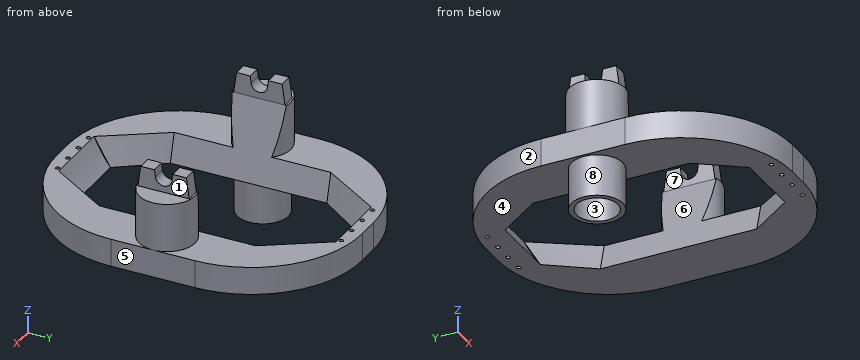
```python
from build123d import *

# Parameters (mm, degrees)
SKETCH_1_R                      = 18.5
SKETCH_1_R_2                    = 15
EXTRUDE_1_DEPTH                 = 30
SKETCH_2_R                      = 20.2
SKETCH_2_R_2                    = 15
EXTRUDE_2_DEPTH                 = 5
SKETCH_3_R                      = 20.2
EXTRUDE_3_DEPTH                 = 50
EXTRUDE_4_DEPTH                 = 5
EXTRUDE_5_DEPTH                 = 20
FILLET_1_R                      = 80
CUT_EXTRUDE_2_REACH             = 174.924
SKETCH_7_R                      = 110
CUT_EXTRUDE_2_DIRECTION_2_REACH = 174.924
SKETCH_11_R                     = 1.5
CUT_EXTRUDE_3_DEPTH             = 25
SKETCH_12_W                     = 57.061720969
SKETCH_12_H                     = 113.011504976
CUT_EXTRUDE_4_DEPTH             = 20


with BuildPart() as part:
    # 草图1 → 凸台-拉伸1 (new body)
    with BuildSketch(Plane.XY):
        Circle(SKETCH_1_R)
        Circle(SKETCH_1_R_2, mode=Mode.SUBTRACT)
    extrude(amount=EXTRUDE_1_DEPTH)

    # 草图2 → 凸台-拉伸2 (add)
    with BuildSketch(Plane.XY.offset(30)):
        Circle(SKETCH_2_R)
        Circle(SKETCH_2_R_2, mode=Mode.SUBTRACT)
    extrude_2 = extrude(amount=EXTRUDE_2_DEPTH)

    # 草图3 → 凸台-拉伸3 (add)
    with BuildSketch(Plane.XY.offset(35)):
        Circle(SKETCH_3_R)
    extrude_3 = extrude(amount=EXTRUDE_3_DEPTH)

    # 草图5 → 凸台-拉伸4 (add, symmetric)
    with BuildSketch(Plane(origin=(0, 0, 0), x_dir=(0, -1, 0), z_dir=(1, 0, 0))):
        with BuildLine():
            Line((-18.5, -85), (18.5, -85))
            Line((18.5, -85), (16.5, -100))
            Line((16.5, -100), (6.5, -100))
            Line((6.5, -100), (5.966081527, -95))
            ThreePointArc((5.966081527, -95), (0, -89.637080228), (-5.966081527, -95))
            Line((-5.966081527, -95), (-6.5, -100))
            Line((-6.5, -100), (-16.5, -100))
            Line((-16.5, -100), (-18.5, -85))
        make_face()
    extrude_4 = extrude(amount=EXTRUDE_4_DEPTH, both=True)

    # 草图6 → 凸台-拉伸5 (add)
    with BuildSketch(Plane(origin=(0, 0, 30), x_dir=(-1, 0, 0), z_dir=(0, 0, -1))):
        Polygon((20.2, 0), (20.2, 110.346509277), (-155.6, 110.346509277), (-155.6, 0), (-155.6, -110.346509277), (20.2, -110.346509277), align=None)
        Polygon((-115.2, 56.505752488), (-92.7, 56.505752488), (-92.7, 85), (-42.7, 85), (-42.7, 56.505752488), (-20.2, 56.505752488), (-20.2, -56.505752488), (-42.7, -56.505752488), (-42.7, -85), (-92.7, -85), (-92.7, -56.505752488), (-115.2, -56.505752488), align=None, mode=Mode.SUBTRACT)
    extrude(amount=-EXTRUDE_5_DEPTH)

    # 镜向1: 凸台-拉伸2, 凸台-拉伸3, 凸台-拉伸4 across plane
    add(extrude_2.mirror(Plane.ZY.offset(-67.7)))
    add(extrude_3.mirror(Plane.ZY.offset(-67.7)))
    add(extrude_4.mirror(Plane.ZY.offset(-67.7)))

    # 圆角1
    fillet_1_edges = [part.edges().sort_by_distance(p)[0] for p in [
        (-20.2, 110.346509277, 40),
        (-20.2, -110.346509277, 40),
        (155.6, -110.346509277, 40),
        (155.6, 110.346509277, 40),
    ]]
    fillet(fillet_1_edges, radius=FILLET_1_R)

    # 切除-拉伸2: up to this face of the body (flat: up to its plane)
    cut_extrude_2_end = Plane(part.part.faces().sort_by_distance((42.7, 70.752876244, 40))[0])
    # 草图7 → 切除-拉伸2 (cut, up to the picked face)
    with BuildSketch(Plane(origin=(67.7, 0, 0), x_dir=(0, 0, -1), z_dir=(1, 0, 0)), mode=Mode.PRIVATE) as cut_extrude_2_sk1:
        with Locations((-95.637080228, 0)):
            Circle(SKETCH_7_R)
    cut_extrude_2_tool1 = split(extrude(cut_extrude_2_sk1.sketch, amount=-CUT_EXTRUDE_2_REACH, mode=Mode.PRIVATE), bisect_by=cut_extrude_2_end, keep=Keep.BOTH, mode=Mode.PRIVATE)
    add(cut_extrude_2_tool1.solids().sort_by(Axis((67.7, 0, 95.63708), (-1, 0, 0)))[0], mode=Mode.SUBTRACT)

    # 切除-拉伸2 direction 2: up to this face of the body (flat: up to its plane)
    cut_extrude_2_direction_2_end = Plane(part.part.faces().sort_by_distance((92.7, 70.752876244, 40))[0])
    # 草图7 → 切除-拉伸2 direction 2 (cut, up to the picked face)
    with BuildSketch(Plane(origin=(67.7, 0, 0), x_dir=(0, 0, -1), z_dir=(1, 0, 0)), mode=Mode.PRIVATE) as cut_extrude_2_direction_2_sk1:
        with Locations((-95.637080228, 0)):
            Circle(SKETCH_7_R)
    cut_extrude_2_direction_2_tool1 = split(extrude(cut_extrude_2_direction_2_sk1.sketch, amount=CUT_EXTRUDE_2_DIRECTION_2_REACH, mode=Mode.PRIVATE), bisect_by=cut_extrude_2_direction_2_end, keep=Keep.BOTH, mode=Mode.PRIVATE)
    add(cut_extrude_2_direction_2_tool1.solids().sort_by(Axis((67.7, 0, 95.63708), (1, 0, 0)))[0], mode=Mode.SUBTRACT)

    # 草图11 → 切除-拉伸3 (cut)
    with BuildSketch(Plane(origin=(0, 0, 30), x_dir=(-1, 0, 0), z_dir=(0, 0, -1))):
        with Locations((-89.646136586, -102.489523561)):
            Circle(SKETCH_11_R)
        with Locations((-75.015378862, -102.489523561)):
            Circle(SKETCH_11_R)
        with Locations((-60.384621138, -102.489523561)):
            Circle(SKETCH_11_R)
        with Locations((-45.753863414, -102.489523561)):
            Circle(SKETCH_11_R)
    cut_extrude_3 = extrude(amount=-CUT_EXTRUDE_3_DEPTH, mode=Mode.SUBTRACT)

    # 镜向2: 切除-拉伸3 across plane
    add(cut_extrude_3.mirror(Plane.ZX), mode=Mode.SUBTRACT)

    # 草图12 → 切除-拉伸4 (cut)
    with BuildSketch(Plane(origin=(26.469269419, 0, 7.315143549), x_dir=(0.26637822592359434, 0, -0.9638685806445808), z_dir=(0.9638685806445808, 0, 0.26637822592359434))):
        with Locations((-52.066077741, 0)):
            Rectangle(SKETCH_12_W, SKETCH_12_H)
    cut_extrude_4 = extrude(amount=CUT_EXTRUDE_4_DEPTH, mode=Mode.SUBTRACT)

    # 镜向3: 切除-拉伸4 across plane
    add(cut_extrude_4.mirror(Plane.ZY.offset(-67.7)), mode=Mode.SUBTRACT)

    # 草图14 → 切除-放样1 section 0
    with BuildSketch(Plane.XY.offset(50)):
        with BuildLine():
            Line((14.672727273, 56.505752488), (42.7, 100.086247348))
            Line((42.7, 100.086247348), (92.7, 100.086247348))
            Line((92.7, 100.086247348), (120.727272727, 56.505752488))
            Line((120.727272727, 56.505752488), (120.727272727, -56.505752488))
            Line((120.727272727, -56.505752488), (92.7, -100.086247348))
            Line((92.7, -100.086247348), (42.7, -100.086247348))
            Line((42.7, -100.086247348), (14.672727273, -56.505752488))
            Line((14.672727273, -56.505752488), (14.672727273, 56.505752488))
        make_face()
    # 草图15 → 切除-放样1 section 1
    with BuildSketch(Plane(origin=(0, 0, 30), x_dir=(-1, 0, 0), z_dir=(0, 0, -1))):
        with BuildLine():
            Line((-92.7, 88.27102412), (-115.2, 56.505752488))
            Line((-115.2, 56.505752488), (-115.2, -56.505752488))
            Line((-115.2, -56.505752488), (-92.7, -88.27102412))
            Line((-92.7, -88.27102412), (-42.7, -88.27102412))
            Line((-42.7, -88.27102412), (-20.2, -56.505752488))
            Line((-20.2, -56.505752488), (-20.2, 56.505752488))
            Line((-20.2, 56.505752488), (-42.7, 88.27102412))
            Line((-42.7, 88.27102412), (-92.7, 88.27102412))
        make_face()
    loft(mode=Mode.SUBTRACT)


solid = part.part
```
Check sheet for the modelled part. Datum: model origin and axes. Units: mm. Face numbers are marked on the shaded views. A direction names the side the tool comes from. Round coordinates to 2 decimals unless told otherwise and drop trailing zeros. Write each loop counter-clockwise with the first axis right and the second up, starting at its lowest first coordinate (ties: lowest second). Pieces come first, ordered by that corner, then holes. Notation, with made-up numbers: (-11.75, 66) -> (22.25, 66) arc R16 cw to (22.25, 76) -> close; hole circle Ø9 at (-33, 61). An arc over 180 degrees is marked (long way). One line per question, with ' | ' between items. Start each with the question number.
1. Sectioned sample at D-D, the plane x = 10. Record the cut outline in (y, z), then the cut area to 3 significant figures.
2. Scan lines: line 1 along Y through (x, z) = (0, 22.75); line 2 along Z through (x, y) = (4, 86.5); line 3 along X through (y, z) = (-54.5, 35). Record each from-to range of solid material in increasing order. Write a range as from..to.
3. Release check for a two-part mould opening along X. For the marked faces 1, 2, 3 and 4 record: +X half, -X half, draft (parallel to the pull), parting line (faces both ways), or undercut.
4. Sectioned sample at C-C, the plane y = 37. Record the cut outline in (x, z).
5. Sectioned sample at A-A, the plane y = 3. Record the cut outline in (x, z), then the cut area to 3 significant figures.
6. Depth check by flat-ended pin: pin 1 (4 mm diameter, centred on x = 11.5, y = -67.5, fed in from -Z); pin 2 (9.5 mm diameter, centred on y = -94.5, z = 39, fed in from -X); pin 3 (13 mm diameter, centred on y = 92, z = 38, fed in from -X). Enter the tip coordinate at first touch or a pass-through.
7. Sectioned sample at B-B, the plane x = 134.5. Record the cut outline in (y, z), then the cut area to 3 significant figures.
8. Set-up check for the marked faces 5, 6, 7 and 8: record each of +Z, -Z, +X, -X, +Y, -Y from which the full face is reachable in a straight line by a thin tool's end or side.
Taken from the geometry:
1) outline: (-92.96, 30) -> (-15.56, 30) -> (-15.56, 0) -> (-11.18, 0) -> (-11.18, 30) -> (11.18, 30) -> (11.18, 0) -> (15.56, 0) -> (15.56, 30) -> (92.96, 30) -> (92.96, 50) -> (17.55, 50) -> (17.55, 66.91) -> (-17.55, 66.91) -> (-17.55, 50) -> (-92.96, 50) -> close | area: 4,570 mm^2
2) line 1: y = -18.5..-15, 15..18.5 | line 2: z = 30..50 | line 3: x = -16.47..18.82, 116.58..151.87
3) face 1: +X half | face 2: -X half | face 3: undercut | face 4: draft
4) outline: (-19.92, 30) -> (20.2, 30) -> (14.67, 50) -> (-19.92, 50) -> close; (115.2, 30) -> (155.32, 30) -> (155.32, 50) -> (120.73, 50) -> close
5) outline: (-20.2, 30) -> (-18.26, 30) -> (-18.26, 0) -> (-14.7, 0) -> (-14.7, 30) -> (14.7, 30) -> (14.7, 0) -> (18.26, 0) -> (18.26, 30) -> (20.2, 30) -> (5, 85) -> (5, 90.44) -> (-5, 90.44) -> (-5, 85) -> (-19.98, 85) -> (-19.98, 50) -> (-20.2, 50) -> close; (115.2, 30) -> (155.6, 30) -> (155.6, 50) -> (155.38, 50) -> (155.38, 85) -> (140.4, 85) -> (140.4, 90.44) -> (130.4, 90.44) -> (130.4, 85) -> close | area: 3,910 mm^2
6) pin 1: stops at z = 30 | pin 2: stops at x = 6.22 | pin 3: stops at x = 1.85
7) outline: (-84.48, 30) -> (84.48, 30) -> (84.48, 50) -> (20.18, 50) -> (20.18, 85) -> (18.5, 85) -> (16.5, 100) -> (6.5, 100) -> (5.97, 95) arc R6 cw to (-5.97, 95) -> (-6.5, 100) -> (-16.5, 100) -> (-18.5, 85) -> (-20.18, 85) -> (-20.18, 50) -> (-84.48, 50) -> close | area: 5,210 mm^2
8) face 5: +Z, -Z, +X, +Y, -Y | face 6: +Z | face 7: +Z, +Y, -Y | face 8: -Z
